Geometry check sheet. Reference: the model listing, model coordinates, mm. A direction names the side the tool comes from. Give positions to 0.01 mm unless a question says otherwise; leave off trailing zeros. Write each loop counter-clockwise with the first axis right and the second up, starting at its lowest first coordinate (ties: lowest second). Pieces come first, ordered by that corner, then holes. Notation, with made-up numbers: (82.5, 14.5) - (116.5, 14.5) arc R20 cw to (116.5, 44.5) - close; hole circle Ø1 at (44.25, -10.75). An arc over 180 degrees is marked (long way). Write item = value, one per line. Start each with the question number.
(1) Access from +Z, -Z, +X, -X, +Y, -Y to the whole of each face (thin tool, end or side, straight path). Record for faces 4 (the flat face through (-4, -18.923, 3)), 5 (the flat face through (2, -10.033, 3)), 6 (the flat face through (-1, 0, 6.477)).
(2) Section check B-B, the plane z = 2. Enter the section's corners in (x, y) (1 decimal), plus the area to 3 significant figures.
(3) Depth check by flat-ended pin: pin 1 Ø0.8 at (x, z) = (-0.5, 2.5) entering from -Y; pin 2 Ø0.6 at (x, z) = (-2, 3) entering from -Y. Enter the tip coordinate at first touch or a pass-through.
(4) Section check A-A, the plane y = 12.7. Enter the section's corners in (x, z).
(5) Draft check along Y on faces 1 (the flat face through (-40.894, 0, 3)), 2 (the cylindrical face through (23.41, 12.8, 3.19)), 3 (the flat face through (0, -6.223, 3)). Enter one of: pulls with the +Y half, pulls with the -Y half, needs draft (parallel to the pull), parting line crosses it, or undercut.
(6) Thickness scan on L1, parallel to X at y = -15, z = 0.75; L2, parallel to X at y = -11, z = 2.25 (3 decimals); L3, parallel to Y at x = 26, z = 3. Record the ranges inside material, lowest first.
```python
from build123d import *

# Parameters (mm, degrees)
SKETCH1_R           = 1.63195
SKETCH1_R_2         = 2.2479
BOSS_EXTRUDE1_DEPTH = 6.477


with BuildPart() as part:
    # Sketch1 → Boss-Extrude1 (new body)
    with BuildSketch(Plane.XY):
        Polygon((-6.985, -18.923), (-1.27, -18.923), (-1.27, -12.573), (-3.175, -12.573), (-3.175, -10.033), (-1.27, -10.033), (-1.27, -6.223), (1.27, -6.223), (1.27, -10.033), (3.175, -10.033), (3.175, -12.573), (1.27, -12.573), (1.27, -18.923), (6.985, -18.923), (6.985, -25.4), (40.894, -25.4), (40.894, 25.4), (-40.894, 25.4), (-40.894, -25.4), (-6.985, -25.4), align=None)
        with Locations((-20.447, -22.1615)):
            Circle(SKETCH1_R, mode=Mode.SUBTRACT)
        with Locations((20.447, -22.1615)):
            Circle(SKETCH1_R, mode=Mode.SUBTRACT)
        with Locations((-25.654, 12.7)):
            Circle(SKETCH1_R_2, mode=Mode.SUBTRACT)
        with Locations((25.654, 12.7)):
            Circle(SKETCH1_R_2, mode=Mode.SUBTRACT)
    extrude(amount=BOSS_EXTRUDE1_DEPTH)


solid = part.part
```
Model answer:
q1.face_4 = +Z, -Z, -Y
q1.face_5 = +Z, -Z
q1.face_6 = +Z, +X, -X, +Y, -Y
q2.outline = (-40.9, -25.4) - (-7, -25.4) - (-7, -18.9) - (-1.3, -18.9) - (-1.3, -12.6) - (-3.2, -12.6) - (-3.2, -10) - (-1.3, -10) - (-1.3, -6.2) - (1.3, -6.2) - (1.3, -10) - (3.2, -10) - (3.2, -12.6) - (1.3, -12.6) - (1.3, -18.9) - (7, -18.9) - (7, -25.4) - (40.9, -25.4) - (40.9, 25.4) - (-40.9, 25.4) - close; hole circle Ø4.5 at (-25.7, 12.7); hole circle Ø3.3 at (-20.4, -22.2); hole circle Ø3.3 at (20.4, -22.2); hole circle Ø4.5 at (25.7, 12.7)
q2.area = 3,970 mm²
q3.pin_1 = -6.22
q3.pin_2 = -18.92
q4.outline = (-40.89, 0) - (-27.9, 0) - (-27.9, 6.48) - (-40.89, 6.48) - close; (-23.41, 0) - (23.41, 0) - (23.41, 6.48) - (-23.41, 6.48) - close; (27.9, 0) - (40.89, 0) - (40.89, 6.48) - (27.9, 6.48) - close
q5.face_1 = needs draft
q5.face_2 = undercut
q5.face_3 = pulls with the -Y half
q6.L1 = -40.89 to -1.27, 1.27 to 40.89
q6.L2 = -40.894 to -3.175, 3.175 to 40.894
q6.L3 = -25.4 to 10.48, 14.92 to 25.4
